Check sheet for the drawn part. Datum: minimum x, y, z corner. Units: mm. Give positions to 0.01 mm unless a question says otherwise; leave off trailing zeros. Order: outer loops, then holes, each group sorted by start corner. A loop starts at its lowest first (then second) coordinate and runs counter-clockwise, first axis right, second up. Notation, with made-up numbers: (39.25, -16) - (91.25, -16) arc R22 cw to (91.25, 17) - close; hole circle Ø5 at (36, 11.5). An arc over 180 degrees is marked (long way). Answer as a JSON object with one key per item and string values. Group by question number.
(1) Section check B-B (z = 2.15). Record the boundary of the cut face in (x, y).
(2) Thickness scan on line 1 (Y direction, x = 50, z = 1.5); line 2 (Y direction, x = 25, z = 2.35); line 3 (Y direction, x = 59, z = 1.1). Record the ranges inside material, lowest first.
(3) Depth check by flat-ended pin: pin 1 Ø1.5 at (y, z) = (64, 3) entering from -X; pin 2 Ø1.5 at (x, z) = (52, 2) entering from -Y. Enter the tip coordinate at first touch or a pass-through.
(4) Section check A-A (x = 50). Record the boundary of the cut face in (y, z).
(5) Section check C-C (y = 25). Record the boundary of the cut face in (x, z), then the cut area to 3 significant figures.
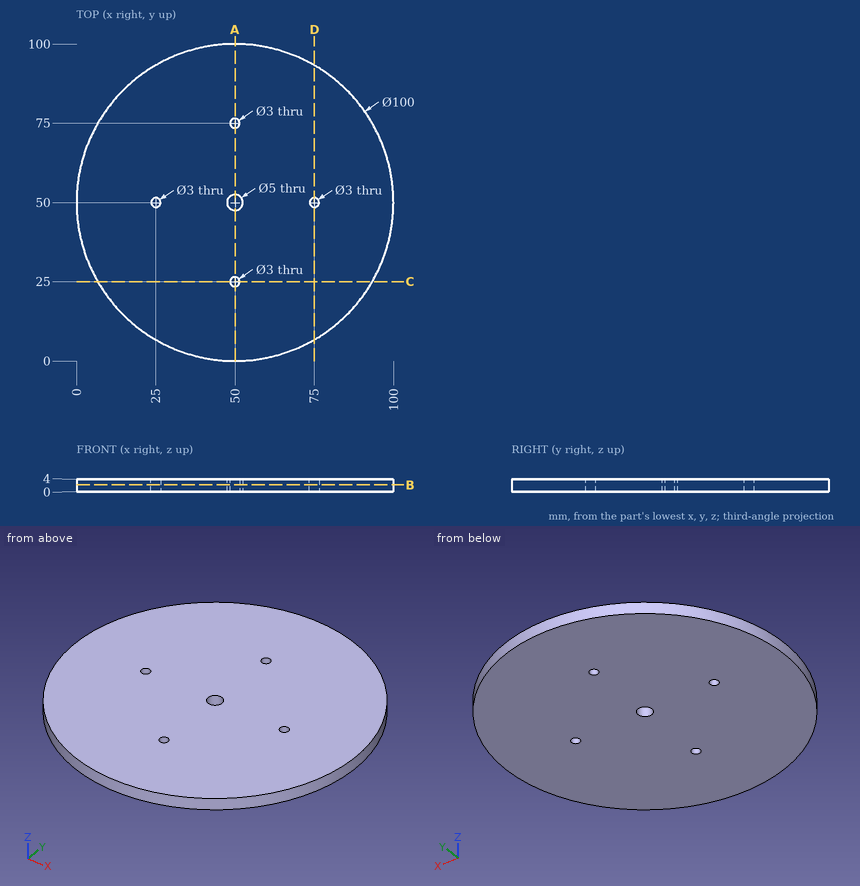
Solutions:
{
 "1": {"outline": "circle Ø100 at (50, 50); hole circle Ø3 at (25, 50); hole circle Ø5 at (50, 50); hole circle Ø3 at (50, 25); hole circle Ø3 at (50, 75); hole circle Ø3 at (75, 50)"},
 "2": {"line 1": "y = 0 to 23.5, 26.5 to 47.5, 52.5 to 73.5, 76.5 to 100", "line 2": "y = 6.7 to 48.5, 51.5 to 93.3", "line 3": "y = 0.82 to 99.18"},
 "3": {"pin 1": "stops at x = 1.79", "pin 2": "stops at y = 0.02"},
 "4": {"outline": "(0, 0) - (23.5, 0) - (23.5, 4) - (0, 4) - close; (26.5, 0) - (47.5, 0) - (47.5, 4) - (26.5, 4) - close; (52.5, 0) - (73.5, 0) - (73.5, 4) - (52.5, 4) - close; (76.5, 0) - (100, 0) - (100, 4) - (76.5, 4) - close"},
 "5": {"outline": "(6.7, 0) - (48.5, 0) - (48.5, 4) - (6.7, 4) - close; (51.5, 0) - (93.3, 0) - (93.3, 4) - (51.5, 4) - close", "area": "334 mm2"}
}
